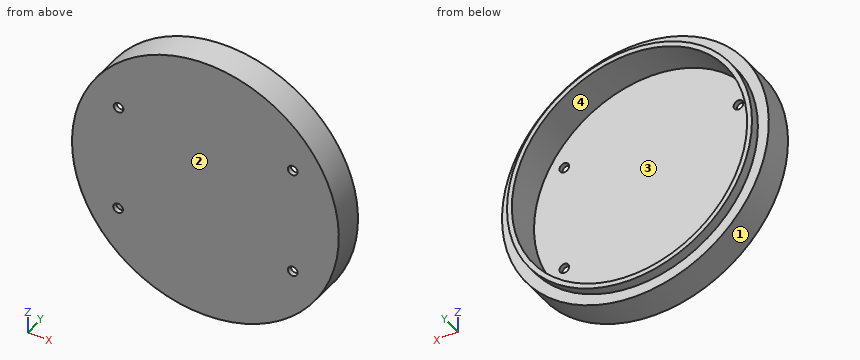
from build123d import *

# Parameters (mm, degrees)
SKETCH2_R           = 55
BOSS_EXTRUDE2_DEPTH = 13
SKETCH7_R           = 50.5
BOSS_EXTRUDE3_DEPTH = 4
SKETCH8_R           = 48.5
CUT_EXTRUDE3_DEPTH  = 15
SKETCH9_R           = 2
CUT_EXTRUDE4_DEPTH  = 15


with BuildPart() as part:
    # Sketch2 → Boss-Extrude2 (new body)
    with BuildSketch(Plane(origin=(0, 0, 0), x_dir=(1, 0, 0), z_dir=(0, 1, 0))):
        with Locations(Location((0, 0, 0), (0, 0, 90))):
            Circle(SKETCH2_R)
    extrude(amount=BOSS_EXTRUDE2_DEPTH)

    # Sketch7 → Boss-Extrude3 (add)
    with BuildSketch(Plane(origin=(0, 13, 0), x_dir=(1, 0, 0), z_dir=(0, 1, 0))):
        with Locations(Location((0, 0, 0), (0, 0, 270))):
            Circle(SKETCH7_R)
    extrude(amount=BOSS_EXTRUDE3_DEPTH)

    # Sketch8 → Cut-Extrude3 (cut)
    with BuildSketch(Plane(origin=(0, 17, 0), x_dir=(1, 0, 0), z_dir=(0, 1, 0))):
        with Locations(Location((0, 0, 0), (0, 0, 270))):
            Circle(SKETCH8_R)
    extrude(amount=-CUT_EXTRUDE3_DEPTH, mode=Mode.SUBTRACT)

    # Sketch9 → Cut-Extrude4 (cut)
    with BuildSketch(Plane(origin=(0, 2, 0), x_dir=(1, 0, 0), z_dir=(0, 1, 0))):
        with Locations(Location((36, -22, 0), (0, 0, 270))):
            Circle(SKETCH9_R)
        with Locations(Location((-36, 22, 0), (0, 0, 270))):
            Circle(SKETCH9_R)
        with Locations(Location((-35.8, -22, 0), (0, 0, 270))):
            Circle(SKETCH9_R)
        with Locations(Location((36, 22, 0), (0, 0, 270))):
            Circle(SKETCH9_R)
    extrude(amount=-CUT_EXTRUDE4_DEPTH, mode=Mode.SUBTRACT)


solid = part.part
Model file for the job. Use its own axes, mm. Face numbers are marked on the shaded views. Coordinates: 2 decimals unless noted, no trailing zeros. Loops run counter-clockwise (first coordinate to the right, second up) from the corner with the lowest first, then second, coordinate; pieces in that order, holes last. Notation, with made-up numbers: (72, -5) -> (90, -5) arc R14 cw to (90, 9) -> close; hole circle Ø7 at (-14.5, -5). An arc over 180 degrees is marked (long way). Use one line per item in the form item = value. Start each with the question number.
(1) Flat gauge pins, fed straight in: pin 1 (2 mm diameter, centred on x = 40, y = 3, fed in from +Z); pin 2 (6 mm diameter, centred on y = 4, z = -19.5, fed in from -X); pin 3 (10 mm diameter, centred on y = 3.5, z = 12.5, fed in from -X). Where does each tip first touch, or does it go through?
(2) Pull direction X, two halves, no side cores. Call the marked faces 1, 2, 3 and 4: pulls with the +X half, pulls with the -X half, needs draft (parallel to the pull), parting line crosses it, or undercut.
(3) Probe probe 1 along X at (y, z) = (9.5, 0); probe 2 along X at (y, z) = (1.4, -22); probe 3 along Y at (x, z) = (29, 38). List the from-to ranges inside material, lowest first. Write a range as from..to.
(4) Cut at B-B on z = 0. Give the cut face in (x, y).
(5) Cut at A-A on x = 36. Give the cut face in (y, z).
(6) Cut at D-D on z = 22. Give the cut face in (x, y), and give its area (3 significant figures).
(7) Cut at C-C on x = 14.5. Give the cut face in (y, z).
Values:
q1.pin_1 = 38.78
q1.pin_2 = -52.47
q1.pin_3 = -54.49
q2.face_1 = parting line crosses it
q2.face_2 = needs draft
q2.face_3 = undercut
q2.face_4 = undercut
q3.probe_1 = -55..-48.5, 48.5..55
q3.probe_2 = -50.41..-38, -34..34, 38..50.41
q3.probe_3 = 0..2
q4.outline = (-55, 0) -> (55, 0) -> (55, 13) -> (50.5, 13) -> (50.5, 17) -> (48.5, 17) -> (48.5, 2) -> (-48.5, 2) -> (-48.5, 17) -> (-50.5, 17) -> (-50.5, 13) -> (-55, 13) -> close
q5.outline = (0, -41.58) -> (13, -41.58) -> (13, -35.42) -> (17, -35.42) -> (17, -32.5) -> (2, -32.5) -> (2, -24) -> (0, -24) -> close; (0, -20) -> (2, -20) -> (2, 20) -> (0, 20) -> close; (0, 24) -> (2, 24) -> (2, 32.5) -> (17, 32.5) -> (17, 35.42) -> (13, 35.42) -> (13, 41.58) -> (0, 41.58) -> close
q6.outline = (-50.41, 0) -> (-37.8, 0) -> (-37.8, 2) -> (-43.22, 2) -> (-43.22, 17) -> (-45.46, 17) -> (-45.46, 13) -> (-50.41, 13) -> close; (-33.8, 0) -> (34, 0) -> (34, 2) -> (-33.8, 2) -> close; (38, 0) -> (50.41, 0) -> (50.41, 13) -> (45.46, 13) -> (45.46, 17) -> (43.22, 17) -> (43.22, 2) -> (38, 2) -> close
q6.area = 362 mm2
q7.outline = (0, -53.05) -> (13, -53.05) -> (13, -48.37) -> (17, -48.37) -> (17, -46.28) -> (2, -46.28) -> (2, 46.28) -> (17, 46.28) -> (17, 48.37) -> (13, 48.37) -> (13, 53.05) -> (0, 53.05) -> close
